from build123d import *

# Parameters (mm, degrees)
F0_R     = 2.15265
F0_R_2   = 3
F0_R_3   = 15.497899
F1_DEPTH = 5.08


with BuildPart() as f1:
    # F0 (on Top) → F1 (new body)
    with BuildSketch(Plane.XY):
        with BuildLine():
            Line((50.8, 92.272936), (-117.584017, 92.272936))
            ThreePointArc((-117.584017, 92.272936), (-120.951629, 90.878016), (-122.346517, 87.510391))
            Line((-122.346517, 87.510391), (-122.345227, -49.059594))
            ThreePointArc((-122.345227, -49.059594), (-120.990568, -52.498598), (-117.584017, -53.932913))
            Line((-117.584017, -53.932913), (50.8, -53.932913))
            Line((50.8, -53.932913), (50.8, 92.272936))
        make_face()
        with Locations((-117.584017, -49.170413)):
            Circle(F0_R, mode=Mode.SUBTRACT)
        with Locations((46.0375, -49.170413)):
            Circle(F0_R, mode=Mode.SUBTRACT)
        with Locations((-27.712823, -16.000006)):
            Circle(F0_R_2, mode=Mode.SUBTRACT)
        Circle(F0_R_3, mode=Mode.SUBTRACT)
        with Locations((27.712823, -16.000006)):
            Circle(F0_R_2, mode=Mode.SUBTRACT)
        with Locations((-117.584017, 87.510436)):
            Circle(F0_R, mode=Mode.SUBTRACT)
        with Locations((0, 32.000012)):
            Circle(F0_R_2, mode=Mode.SUBTRACT)
        with Locations((46.0375, 87.510436)):
            Circle(F0_R, mode=Mode.SUBTRACT)
    extrude(amount=F1_DEPTH)


solid = f1.part
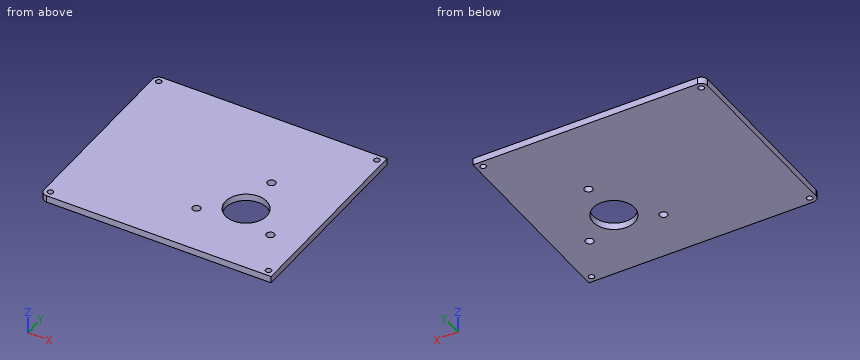
Geometry check sheet. Reference: the model listing, model coordinates, mm. Give positions to 0.01 mm unless a question says otherwise; leave off trailing zeros. Loops run counter-clockwise (first coordinate to the right, second up) from the corner with the lowest first, then second, coordinate; pieces in that order, holes last. Notation, with made-up numbers: (86, 5) -> (96, 5) arc R14 ccw to (96, 24) -> close; hole circle Ø1 at (-38.5, 48). An arc over 180 degrees is marked (long way). Answer in a Markdown table with one row per item. Add a question column.
1) Cross-section at A-A on x = 0. Record the boundary of the cut face in (y, z).
2) Material ranges on probe 1 along X at (y, z) = (-16, 0.95); probe 2 along X at (y, z) = (-17, 1.85); probe 3 along X at (y, z) = (-37.5, 1.3), recorded low to high. Write a range as from..to.
3) Cross-section at B-B on y = 0. Record the boundary of the cut face in (x, z), and give its area (3 significant figures).
4) Cross-section at C-C on z = 1.4. State how many separate pieces and enclosed holes the cut face has, and give its area (3 significant figures).
Outcome:
| question | item | result |
|---|---|---|
| 1 | outline | (-53.93, 0) -> (-15.5, 0) -> (-15.5, 5.08) -> (-53.93, 5.08) -> close; (15.5, 0) -> (29, 0) -> (29, 5.08) -> (15.5, 5.08) -> close; (35, 0) -> (92.27, 0) -> (92.27, 5.08) -> (35, 5.08) -> close |
| 2 | probe 1 | x = -122.35..-30.71, -24.71..24.71, 30.71..50.8 |
| 2 | probe 2 | x = -122.35..-30.54, -24.88..24.88, 30.54..50.8 |
| 2 | probe 3 | x = -122.35..50.8 |
| 3 | outline | (-122.35, 0) -> (-15.5, 0) -> (-15.5, 5.08) -> (-122.35, 5.08) -> close; (15.5, 0) -> (50.8, 0) -> (50.8, 5.08) -> (15.5, 5.08) -> close |
| 3 | area | 722 mm^2 |
| 4 | separate pieces | 1 |
| 4 | enclosed holes | 8 |
| 4 | area | 24,400 mm^2 |
